Geometry check sheet. Reference: the model listing, model coordinates, mm. A direction names the side the tool comes from. Coordinates: 2 decimals unless noted, no trailing zeros. Write each loop counter-clockwise with the first axis right and the second up, starting at its lowest first coordinate (ties: lowest second). Pieces come first, ordered by that corner, then holes.
from build123d import *

# Parameters (mm, degrees)
EXTRUS_O1_DEPTH       = 6
ESBO_O2_R             = 3.5
CORTE_EXTRUS_O1_DEPTH = 12


with BuildPart() as part:
    # Esboço1 → Extrusão1 (new, symmetric)
    with BuildSketch(Plane.XY):
        with BuildLine():
            Line((-10, -0.5), (-10, 0))
            Line((-10, 0), (-2.25, 0))
            ThreePointArc((-2.25, 0), (0, 2.25), (2.25, 0))
            Line((2.25, 0), (3, 0))
            Line((3, 0), (3, 4))
            Line((3, 4), (-12, 4))
            Line((-12, 4), (-12, -0.5))
            Line((-12, -0.5), (-10, -0.5))
        make_face()
    extrude(amount=EXTRUS_O1_DEPTH, both=True)

    # Esboço2 → Corte-extrusão1 (cut)
    with BuildSketch(Plane.XZ):
        with Locations((-6.125, 0)):
            Circle(ESBO_O2_R)
    extrude(amount=-CORTE_EXTRUS_O1_DEPTH, mode=Mode.SUBTRACT)


solid = part.part
1. Sectioned sample at B-B, the plane z = 0. Record the boundary of the cut face in (x, y) (3 decimals), and give its area (3 significant figures).
Computed values:
outline: (-12, -0.5) - (-10, -0.5) - (-10, 0) - (-9.625, 0) - (-9.625, 4) - (-12, 4) - close; (-2.625, 0) - (-2.25, 0) arc R2.25 cw to (2.25, 0) - (3, 0) - (3, 4) - (-2.625, 4) - close
area: 25.0 mm2
2. Sectioned sample at D-D, the plane y = 2.95. Record the boundary of the cut face in (x, z) (3 decimals), and give its area (3 significant figures).
Computed values:
outline: (-12, -6) - (3, -6) - (3, 6) - (-12, 6) - close; hole circle Ø7 at (-6.125, 0)
area: 142 mm2
3. Gauge pin test, flat ends, axial feed: pin 1 Ø5.5 at (x, z) = (-6.125, 0) entering from -Y (3 decimals); pin 2 Ø0.8 at (x, z) = (2.5, 2.5) entering from -Y. Record the tip position at first contact, or that the pin passes through.
Computed values:
pin 1: passes through
pin 2: stops at y = 0
4. Thickness scan on line 1 along Z through (x, y) = (-6.25, 0.95); line 2 along X through (y, z) = (0.05, 3); line 3 along Z through (x, y) = (-8, 3.5). Record the ranges inside material, lowest first.
Computed values:
line 1: z = -6 to -3.5, 3.5 to 6
line 2: x = -12 to -7.93, -4.32 to -2.25, 2.25 to 3
line 3: z = -6 to -2.96, 2.96 to 6
5. Sectioned sample at A-A, the plane y = 1.5. Record the boundary of the cut face in (x, z) (3 decimals).
Computed values:
outline: (-12, -6) - (-1.677, -6) - (-1.677, 6) - (-12, 6) - close; (1.677, -6) - (3, -6) - (3, 6) - (1.677, 6) - close; hole circle Ø7 at (-6.125, 0)
6. Access from +Z, -Z, +X, -X, +Y, -Y to the whole of each face (thin tool, end or side, straight path). Record for faces 5 (the flat face through (-2.7, 0, 1.4)), 6 (the flat face through (-6, 2, 6)).
Computed values:
face 5: +Z, -Z, +X, -Y
face 6: +Z, +X, -X, +Y, -Y
7. Sectioned sample at C-C, the plane z = 4. Record the boundary of the cut face in (x, y), and give its area (3 significant figures).
Computed values:
outline: (-12, -0.5) - (-10, -0.5) - (-10, 0) - (-2.25, 0) arc R2.25 cw to (2.25, 0) - (3, 0) - (3, 4) - (-12, 4) - close
area: 53.0 mm2
8. Draft check along X on faces 1 (the flat face through (-6, 2, -6)), 2 (the cylindrical face through (-6.884, 1.972, -3.417)), 3 (the flat face through (3, 2, 0)), 4 (the cylindrical face through (-0.05, 2.25, 0.08)). Enter one of: released by +X, released by -X, zero draft, split by the parting line, or undercut.
Computed values:
face 1: zero draft
face 2: undercut
face 3: released by +X
face 4: undercut
